Verification items for the finished model (mm, model axes). A direction names the side the tool comes from. Give positions to 0.01 mm unless a question says otherwise; leave off trailing zeros. Loops run counter-clockwise (first coordinate to the right, second up) from the corner with the lowest first, then second, coordinate; pieces in that order, holes last. Notation, with made-up numbers: (82, 32) -> (118, 32) arc R22 cw to (118, 62) -> close; hole circle Ø6 at (28.25, -22). An arc over 180 degrees is marked (long way). Answer in a Markdown table with one row per item. Add a question column.
Q1. Set-up check for faces 4 (the face through (422.55, 102.13, 6.44)), 5 (the face through (60, 25.4, 10)), 6 (the face through (405.39, 19, 13)), 7 (the face through (500.38, 36, 13)): record each of +Z, -Z, +X, -X, +Y, -Y from which the full face is reachable in a straight line by a thin tool's end or side.
Q2. Section check B-B on x = 153. Enter the section's corners in (y, z), and give its area (3 significant figures).
Q3. Release check for a two-part mould opening along Z. For faces 1 (the face through (184, 25.4, 10)), 2 (the face through (350, 51, 12.7)), 3 (the face through (470.76, 90.43, 12.61)) record: pulls with the +Z half, pulls with the -Z half, needs draft (parallel to the pull), parting line crosses it, or undercut.
Q4. Gauge pin test, flat ends, axial feed: P1, Ø1.2, axis at y = 80, z = 12, coming from the +X side; P2, Ø3, axis at x = 465, z = 13.5, coming from the -Y side; P3, Ø1.5, axis at x = 457, z = 8, coming from the +Y side. Record the tip position at first contact, or that the pin passes through.
Q5. Material ranges on probe 1 along Y at (x, z) = (478, 12.7); probe 2 along X at (y, z) = (22, 5.5); probe 3 along X at (y, z) = (26, 1.75), recorded low to high.
Q6. Section check A-A on y = 130. Enter the section's corners in (x, z), and give its area (3 significant figures).
Q7. Section check C-C on y = 204. Give the number of separate pieces and of enclosed holes in the cut face, and give its area (3 significant figures).
Autodesk Inventor part; units mm, degrees
ref_plane "YZ Plane" through (0, 0, 0) normal (1, 0, 0) x (0, 1, 0)
ref_plane "XZ Plane" through (0, 0, 0) normal (0, 1, 0) x (-1, 0, 0)
ref_plane "XY Plane" through (0, 0, 0) normal (0, 0, 1) x (1, 0, 0)
sketch "Sketch1" plane through (0, 0, 0) normal (0, 0, 1) x (1, 0, 0)
  line L0 (262.89, 253.3796) -> (525.78, 101.6)
  line L1 (525.78, 101.6) -> (525.78, -201.9592) construction
  line L2 (525.78, -201.9592) -> (262.89, -353.7388) construction
  line L3 (262.89, -353.7388) -> (0, -201.9592) construction
  line L4 (0, -201.9592) -> (0, 101.6) construction
  line L5 (0, 101.6) -> (262.89, 253.3796)
  line L6 (0, 101.6) -> (0, 0)
  line L7 (0, 0) -> (525.78, 0)
  line L8 (525.78, 0) -> (525.78, 101.6)
  point P0 (262.89, -50.1796)
  dimension "d0" = 525.78
  dimension "d1" = 101.6
extrude "Extrusion1" add sketch "Sketch1" along normal blind 25.4
sketch "Sketch2" plane through (0, 0, 25.4) normal (0, 0, 1) x (1, 0, 0)
  circle A0 centre (262.89, 121.3796) radius 22.5
  line L0 (0, 0) -> (525.78, 0)
  point P0 (262.89, 0)
  dimension "d4" = 121.3796
  dimension "d5" = 45
extrude "Extrusion2" cut sketch "Sketch2" against normal through all
sketch "Sketch3" plane through (0, 0, 25.4) normal (0, 0, 1) x (1, 0, 0)
  circle A0 centre (262.89, 121.3796) radius 22.5
  line L0 (0, 101.6) -> (0, 0)
  line L1 (0, 0) -> (525.78, 0)
  line L2 (525.78, 0) -> (525.78, 101.6)
  line L3 (525.78, 101.6) -> (262.89, 253.3796)
  line L4 (262.89, 253.3796) -> (0, 101.6)
  line L5 (25.4, 86.9353) -> (25.4, 25.4)
  line L6 (25.4, 25.4) -> (500.38, 25.4)
  line L7 (500.38, 25.4) -> (500.38, 86.9353)
  line L8 (500.38, 86.9353) -> (262.89, 224.0502)
  line L9 (262.89, 224.0502) -> (25.4, 86.9353)
  dimension "d8" = 25.4
extrude "Extrusion3" cut sketch "Sketch3" against normal through all contours L4 L3 L2 L1 L0
sketch "Sketch4" plane through (0, 0, 25.4) normal (0, 0, 1) x (1, 0, 0)
  line L0 (134.346, 149.8353) -> (159.746, 105.8412)
  line L1 (159.746, 105.8412) -> (115.7519, 80.4412)
  line L2 (115.7519, 80.4412) -> (90.3519, 124.4353)
  line L3 (90.3519, 124.4353) -> (134.346, 149.8353)
  line L4 (134.346, 149.8353) -> (115.7519, 80.4412) construction
  line L5 (159.746, 105.8412) -> (90.3519, 124.4353) construction
  line L6 (262.89, 224.0502) -> (25.4, 86.9353)
  line L7 (500.38, 86.9353) -> (262.89, 224.0502)
  line L8 (262.89, 224.0502) -> (262.89, 25.4)
  line L9 (25.4, 25.4) -> (500.38, 25.4)
  line L10 (391.434, 149.8353) -> (366.034, 105.8412)
  line L11 (366.034, 105.8412) -> (410.0281, 80.4412)
  line L12 (410.0281, 80.4412) -> (435.4281, 124.4353)
  line L13 (435.4281, 124.4353) -> (391.434, 149.8353)
  line L14 (391.434, 149.8353) -> (410.0281, 80.4412) construction
  line L15 (366.034, 105.8412) -> (435.4281, 124.4353) construction
  point P0 (0, 0)
  point P1 (125.049, 115.1383)
  point P2 (400.731, 115.1383)
  point P3 (381.635, 155.4928)
  dimension "d11" = 50.8
  dimension "d12" = 50.8
  dimension "d15" = 75
extrude "Extrusion4" cut sketch "Sketch4" against normal through all
sketch "Sketch5" plane through (0, 0, 0) normal (0, 0, -1) x (-1, 0, 0)
  line L0 (-25.4, 86.9353) -> (-25.4, 25.4)
  line L1 (-25.4, 43.4677) -> (-12.7, 43.4677)
  line L2 (-12.7, 43.4677) -> (-12.7, 68.8677)
  line L3 (-12.7, 68.8677) -> (-25.4, 68.8677)
  line L4 (-25.4, 68.8677) -> (-25.4, 43.4677)
  line L5 (-25.4, 25.4) -> (-500.38, 25.4)
  line L6 (-94.99, 25.4) -> (-120.39, 25.4)
  line L7 (-120.39, 25.4) -> (-120.39, 12.7)
  line L8 (-120.39, 12.7) -> (-94.99, 12.7)
  line L9 (-94.99, 12.7) -> (-94.99, 25.4)
  line L10 (-405.39, 25.4) -> (-430.79, 25.4)
  line L11 (-430.79, 25.4) -> (-430.79, 12.7)
  line L12 (-430.79, 12.7) -> (-405.39, 12.7)
  line L13 (-405.39, 12.7) -> (-405.39, 25.4)
  line L14 (-500.38, 25.4) -> (-500.38, 86.9353)
  line L15 (-500.38, 43.4677) -> (-513.08, 43.4677)
  line L16 (-513.08, 43.4677) -> (-513.08, 68.8677)
  line L17 (-513.08, 68.8677) -> (-500.38, 68.8677)
  line L18 (-500.38, 68.8677) -> (-500.38, 43.4677)
  line L19 (-262.89, 224.0502) -> (-134.346, 149.8353)
  line L20 (-198.618, 186.9428) -> (-220.615, 199.6428)
  line L21 (-220.615, 199.6428) -> (-214.265, 210.6413)
  line L22 (-214.265, 210.6413) -> (-192.268, 197.9413)
  line L23 (-192.268, 197.9413) -> (-198.618, 186.9428)
  line L24 (-391.434, 149.8353) -> (-262.89, 224.0502)
  line L25 (-305.165, 199.6428) -> (-327.162, 186.9428)
  line L26 (-327.162, 186.9428) -> (-333.512, 197.9413)
  line L27 (-333.512, 197.9413) -> (-311.515, 210.6413)
  line L28 (-311.515, 210.6413) -> (-305.165, 199.6428)
  line L29 (-262.89, 224.0502) -> (-391.434, 149.8353)
  line L30 (-120.39, 19.05) -> (-405.39, 19.05) construction
  line L31 (-250.19, 25.4) -> (-275.59, 25.4)
  line L32 (-275.59, 25.4) -> (-275.59, 12.7)
  line L33 (-275.59, 12.7) -> (-250.19, 12.7)
  line L34 (-250.19, 12.7) -> (-250.19, 25.4)
  line L35 (-500.38, 25.4) -> (-25.4, 25.4)
  line L36 (-305.165, 199.6428) -> (-311.515, 210.6413)
  line L37 (-311.515, 210.6413) -> (-333.512, 197.9413)
  line L38 (-333.512, 197.9413) -> (-327.162, 186.9428)
  line L39 (-327.162, 186.9428) -> (-305.165, 199.6428)
  point P0 (0, 0)
  point P1 (-25.4, 56.1677)
  point P2 (-262.89, 25.4)
  point P3 (-262.89, 19.05)
  point P4 (-262.89, 25.4)
  dimension "d16" = 12.7
  dimension "d17" = 12.7
  dimension "d18" = 12.7
  dimension "d19" = 12.7
  dimension "d20" = 12.7
  dimension "d21" = 12.7
  dimension "d22" = 25.4
  dimension "d23" = 25.4
  dimension "d24" = 25.4
  dimension "d25" = 25.4
  dimension "d26" = 25.4
  dimension "d27" = 25.4
  dimension "d28" = 285
  dimension "d29" = 25.4
  dimension "d30" = 12.7
extrude "Extrusion5" add sketch "Sketch5" against normal blind 25.4
sketch "Sketch6" plane through (0, 0, 0) normal (0, 0, -1) x (-1, 0, 0)
  line L0 (-275.59, 25.4) -> (-405.39, 25.4)
  line L1 (-324.58, 25.4) -> (-375.38, 25.4)
  line L2 (-375.38, 25.4) -> (-375.38, 76.2)
  line L3 (-375.38, 76.2) -> (-324.58, 76.2)
  line L4 (-324.58, 76.2) -> (-324.58, 25.4)
  line L5 (-500.38, 43.4677) -> (-500.38, 25.4)
  point P0 (0, 0)
  dimension "d33" = 50.8
  dimension "d34" = 50.8
  dimension "d35" = 125
extrude "Extrusion6" cut sketch "Sketch6" against normal blind 12.7
sketch "Sketch7" plane through (0, 0, 25.4) normal (0, 0, 1) x (1, 0, 0)
  line L0 (115.2118, 50.8) -> (183.4445, 90.1942)
  line L1 (183.4445, 90.1942) -> (206.1888, 50.8)
  line L2 (206.1888, 50.8) -> (115.2118, 50.8)
  line L3 (159.746, 105.8412) -> (115.7519, 80.4412)
  line L4 (120.39, 25.4) -> (250.19, 25.4)
  line L5 (134.346, 149.8353) -> (159.746, 105.8412)
  point P0 (0, 0)
  dimension "d39" = 25.4
  dimension "d40" = 25.4
  dimension "d41" = 12.7
extrude "Extrusion7" cut sketch "Sketch7" against normal through all
sketch "Sketch8" plane through (0, 0, 25.4) normal (0, 0, 1) x (1, 0, 0)
  circle A0 centre (307.0573, 146.8796) radius 2.5
  circle A1 centre (262.89, 121.3796) radius 22.5
  circle A2 centre (262.89, 172.3796) radius 2.5
  circle A3 centre (218.7227, 146.8796) radius 2.5
  circle A4 centre (218.7227, 95.8796) radius 2.5
  circle A5 centre (262.89, 70.3796) radius 2.5
  circle A6 centre (307.0573, 95.8796) radius 2.5
  point P0 (0, 0)
  dimension "d44" = 5
  dimension "d48" = 360
  dimension "d56" = 51
extrude "Extrusion8" cut sketch "Sketch8" against normal through all
sketch "Sketch10" plane through (0, 0, 25.4) normal (0, 0, 1) x (1, 0, 0)
  line L0 (115.7519, 80.4412) -> (90.3519, 124.4353)
  line L1 (366.034, 105.8412) -> (391.434, 149.8353)
  line L2 (410.0281, 80.4412) -> (435.4281, 124.4353)
  line L3 (391.434, 149.8353) -> (435.4281, 124.4353)
  line L4 (410.0281, 80.4412) -> (366.034, 105.8412)
  line L5 (134.346, 149.8353) -> (159.746, 105.8412)
  line L6 (159.746, 105.8412) -> (115.7519, 80.4412)
  line L7 (134.346, 149.8353) -> (198.618, 186.9428)
  line L8 (90.3519, 124.4353) -> (134.346, 149.8353)
  point P0 (0, 0)
extrude "Extrusion10" add sketch "Sketch10" against normal blind 12.7
sketch "Sketch11" plane through (500.38, 86.9353, 25.4) normal (0.5, 0.866, 0) x (0.866, -0.5, 0)
  circle A0 centre (-25.4, 12.7) radius 2
  circle A1 centre (-248.8298, 12.7) radius 2
  line L0 (-274.2298, 0) -> (-274.2298, 25.4)
  line L1 (0, 0) -> (0, 25.4)
  point P0 (-389.8741, 25.4)
  point P1 (-274.2298, 12.7)
  dimension "d57" = 4
  dimension "d58" = 4
  dimension "d59" = 25.4
  dimension "d60" = 25.4
extrude "Extrusion11" cut sketch "Sketch11" against normal blind 38.1
sketch "Sketch12" plane through (25.4, 86.9353, 25.4) normal (-0.5, 0.866, 0) x (0.866, 0.5, 0)
  circle A0 centre (248.8298, 12.7) radius 2
  circle A1 centre (25.4, 12.7) radius 2
  line L0 (0, 0) -> (0, 25.4)
  line L1 (274.2298, 0) -> (274.2298, 25.4)
  point P0 (-65.4647, 25.4)
  point P1 (0, 12.7)
  dimension "d63" = 4
  dimension "d64" = 4
  dimension "d65" = 25.4
  dimension "d66" = 25.4
extrude "Extrusion12" cut sketch "Sketch12" against normal blind 38.1
sketch "Sketch13" plane through (500.38, 25.4, 25.4) normal (1, 0, 0) x (0, 0, -1)
  circle A0 centre (12.7, 8) radius 2
  circle A1 centre (12.7, 53.5353) radius 2
  line L0 (0, 0) -> (25.4, 0)
  line L1 (0, 61.5353) -> (25.4, 61.5353)
  point P0 (25.4, -25.4)
  point P1 (12.7, 0)
  point P2 (12.7, 61.5353)
  dimension "d69" = 4
  dimension "d70" = 4
  dimension "d71" = 8
  dimension "d72" = 8
extrude "Extrusion13" cut sketch "Sketch13" against normal blind 38.1
sketch "Sketch14" plane through (25.4, 25.4, 0) normal (-1, 0, 0) x (0, 0, 1)
  circle A0 centre (12.7, 53.5353) radius 2
  circle A1 centre (12.7, 8) radius 2
  point P0 (0, -25.4)
extrude "Extrusion14" cut sketch "Sketch14" against normal blind 38.1
sketch "Sketch15" plane through (120.39, 25.4, 25.4) normal (0, -1, 0) x (1, 0, 0)
  circle A0 centre (-60.195, -12.7) radius 2
  circle A1 centre (64.9, -12.7) radius 2
  circle A2 centre (345.195, -12.7) radius 2
  line L0 (-94.99, 0) -> (-25.4, 0)
  line L1 (310.4, 0) -> (379.99, 0)
  line L2 (-94.99, 0) -> (-94.99, -25.4)
  line L3 (0, 0) -> (129.8, 0)
  point P0 (-120.39, -25.4)
  point P1 (-60.195, 0)
  point P2 (345.195, 0)
  point P3 (-94.99, -12.7)
  point P4 (64.9, 0)
  dimension "d77" = 4
  dimension "d78" = 4
  dimension "d79" = 4
extrude "Extrusion15" cut sketch "Sketch15" against normal blind 38.1
properties part number "HB04" material "Polyethylene, High Density"
Taken from the geometry:
| question | item | result |
|---|---|---|
| 1 | face 4 | -Z, +Y |
| 1 | face 5 | +Z, -Z, -X, -Y |
| 1 | face 6 | +Z, -Z, -Y |
| 1 | face 7 | +Z, -Z, +X, -Y |
| 2 | outline | (25.4, 0) -> (50.8, 0) -> (50.8, 25.4) -> (25.4, 25.4) -> close; (72.62, 0) -> (101.95, 0) -> (101.95, 12.7) -> (117.53, 12.7) -> (117.53, 0) -> (160.61, 0) -> (160.61, 25.4) -> (72.62, 25.4) -> close |
| 2 | area | 2,680 mm² |
| 3 | face 1 | needs draft |
| 3 | face 2 | pulls with the -Z half |
| 3 | face 3 | undercut |
| 4 | P1 | stops at x = 462.28 |
| 4 | P2 | stops at y = 25.4 |
| 4 | P3 | stops at y = 112.41 |
| 5 | probe 1 | y = 25.4 to 31.4, 35.4 to 76.94, 80.94 to 94.97 |
| 5 | probe 2 | x = 94.99 to 120.39, 250.19 to 275.59, 405.39 to 430.79 |
| 5 | probe 3 | x = 25.4 to 324.58, 375.38 to 500.38 |
| 6 | outline | (99.99, 12.7) -> (145.8, 12.7) -> (145.8, 0) -> (242.11, 0) -> (242.11, 25.4) -> (99.99, 25.4) -> close; (283.67, 0) -> (379.98, 0) -> (379.98, 12.7) -> (425.79, 12.7) -> (425.79, 25.4) -> (283.67, 25.4) -> close |
| 6 | area | 6,060 mm² |
| 7 | separate pieces | 3 |
| 7 | enclosed holes | 2 |
| 7 | area | 2,510 mm² |
